Can you work these out from the drawing? Everything is in mm from the part's minimum corner. A direction names the side the tool comes from. Round coordinates to 2 decimals unless told otherwise and drop trailing zeros. Order: outer loops, then holes, each group sorted by start corner. A loop starts at its lowest first (then second) coordinate and runs counter-clockwise, first axis right, second up. Notation, with made-up numbers: (70, 30.25) - (106, 30.25) arc R24 ccw to (106, 44.25) - close; hole circle Ø7 at (48, 35). An arc over 180 degrees is marked (long way). Answer as a JSON object with one key per item and string values.
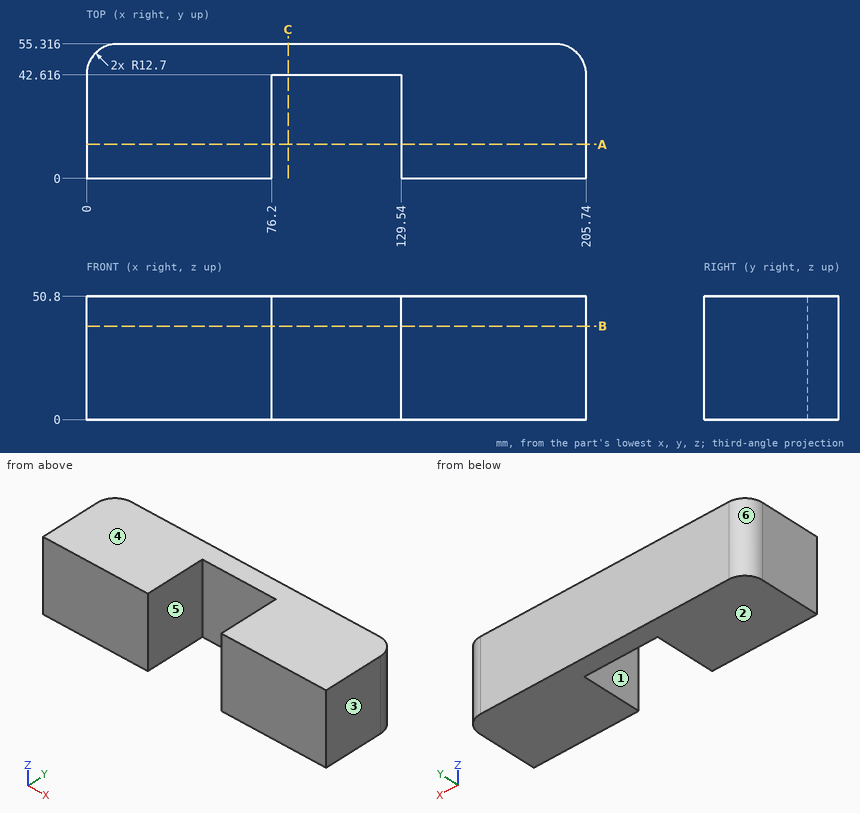
1. Imagine slicing it at A-A (y = 14). List the corners of the cut face in (x, z) for me, plus the area to 3 significant figures.
Responses:
{"outline": "(0, 0) - (76.2, 0) - (76.2, 50.8) - (0, 50.8) - close; (129.54, 0) - (205.74, 0) - (205.74, 50.8) - (129.54, 50.8) - close", "area": "7,740 mm2"}
2. For P1, Ø5, axis at x = 107.5, z = 17.5, coming from the -Y side, with a flat end and sliding along its axis, tell me the tip position at first contact or that it passes through.
Responses:
{"P1": "y = 42.62"}
3. Thinking about a two-plate mould opening in X: for the marked faces 3, 4, 5 and 6, which applies, pulls with the +X half, pulls with the -X half, needs draft (parallel to the pull), parting line crosses it, or undercut?
Responses:
{"face 3": "pulls with the +X half", "face 4": "needs draft", "face 5": "undercut", "face 6": "pulls with the -X half"}
4. Imagine slicing it at B-B (z = 38.5). List the corners of the cut face in (x, y) for me, plus the area to 3 significant figures.
Responses:
{"outline": "(0, 0) - (76.2, 0) - (76.2, 42.62) - (129.54, 42.62) - (129.54, 0) - (205.74, 0) - (205.74, 42.62) arc R12.7 ccw to (193.04, 55.32) - (12.7, 55.32) arc R12.7 ccw to (0, 42.62) - close", "area": "9,040 mm2"}
5. Imagine slicing it at C-C (x = 83). List the corners of the cut face in (y, z) for me.
Responses:
{"outline": "(42.62, 0) - (55.32, 0) - (55.32, 50.8) - (42.62, 50.8) - close"}
6. For the marked faces 1 and 2, which set-ups out of +Z, -Z, +X, -X, +Y, -Y let a thin tool reach every point of the face, with its end or its side?
Responses:
{"face 1": "+Z, -Z, -Y", "face 2": "-Z, +X, -X, +Y, -Y"}
7. If I drill on L1, parallel to X at y = 6, z = 41.5; L2, parallel to Y at x = 118.5, z = 23.5; L3, parallel to X at y = 43, z = 31, over which ranges is the centre line in solid material (lowest first)? Write a range as [from, to].
Responses:
{"L1": "[0, 76.2], [129.54, 205.74]", "L2": "[42.62, 55.32]", "L3": "[0.01, 205.73]"}
